The model under review builds one solid part; all positions refer to its coordinate system, in mm. A direction names the side the tool comes from. Coordinates: 2 decimals unless noted, no trailing zeros. Write each loop counter-clockwise with the first axis right and the second up, starting at its lowest first coordinate (ties: lowest second). Pieces come first, ordered by that corner, then holes.
1) For P1, Ø2, axis at y = 13.5, z = -2, coming from the +X side; P2, Ø12, axis at x = 7, z = 12, coming from the -Y side; P3, Ø4, axis at x = 8, z = -10.5, coming from the -Y side; P4, Ø4, axis at y = -8, z = 6, coming from the +X side, all flat-tipped, find the tip position at first contact; note any pin that passes through.
2) For line 1 (Z direction, x = 15, y = 4.5); line 2 (Y direction, x = -4, z = -11.5); line 3 (Z direction, x = -11, y = 13.5), list the stretches that pass through material, from the lowest coordinate up.
3) Mouldability with a two-part tool opening along X and no side actions: class faces 4 (the cylindrical face through (3.226, 8.018, 13.109)), 5 (the flat face through (-4, 17.144, 0)), 6 (the cylindrical face through (-13.4, 8.02, -1.63)) as released by +X, released by -X, zero draft, split by the parting line, or undercut.
4) Add section B-B, the plane z = 5.5. State the section outline as (x, y) points.
5) Machinability: for faces 1 (the cylindrical face through (10.74, -10.72, -2.38)), 2 (the cylindrical face through (-8.96, 8.02, 10.1)), 3 (the cylindrical face through (0.9, 8.02, 2.86)), which of the approach directions +Z, -Z, +X, -X, +Y, -Y give a long, thin tool a straight path to every point of the face, cutting with its end or side? Answer none if there is none.
6) Add section C-C, the plane y = -15. State the section outline as (x, z) points.
7) Add section A-A, the plane x = 0. State the section outline as (y, z) points, then the cut area to 3 significant figures.
from build123d import *

# Parameters (mm, degrees)
SKETCH1_R           = 1.5
BOSS_EXTRUDE1_DEPTH = 9
SKETCH2_R           = 5.5
BOSS_EXTRUDE2_DEPTH = 10
L_EK2_SCALE         = 2


with BuildPart() as part:
    # Sketch1 → Boss-Extrude1 (new body)
    with BuildSketch(Plane(origin=(0, 0, 0), x_dir=(1, 0, 0), z_dir=(0, 1, 0))):
        with BuildLine():
            add(Edge.make_bspline(
                [(-5.065227978, 4.461610195), (-5.526615005, 4.86619147), (-5.830003112, 5.39406146), (-5.975392301, 6.045220165)],
                knots=[0, 0, 0, 0, 0.872429449, 0.872429449, 0.872429449, 0.872429449], degree=3))
            ThreePointArc((-5.065227978, 4.461610195), (-5.560258819, 3.827012132), (-5.976238464, 3.138004752))
            add(Edge.make_bspline(
                [(-7.780961116, 3.42149735), (-7.125870497, 3.507536778), (-6.52429628, 3.413039245), (-5.976238464, 3.138004752)],
                knots=[0.127683247, 0.127683247, 0.127683247, 0.127683247, 1, 1, 1, 1], degree=3))
            ThreePointArc((-7.780961116, 3.42149735), (-7.951879756, 3.00293329), (-8.10030101, 2.575873357))
            add(Edge.make_bspline(
                [(-6.558450277, 1.596630818), (-7.155006493, 1.740452504), (-7.668956737, 2.066866683), (-8.10030101, 2.575873357)],
                knots=[0, 0, 0, 0, 0.872429449, 0.872429449, 0.872429449, 0.872429449], degree=3))
            ThreePointArc((-6.558450277, 1.596630818), (-6.701865893, 0.804669837), (-6.749999881, 0.00126872))
            add(Edge.make_bspline(
                [(-8.479748007, -0.586407486), (-7.939678588, -0.205787566), (-7.363095879, -0.009895497), (-6.749999881, 0.00126872)],
                knots=[0.127683247, 0.127683247, 0.127683247, 0.127683247, 1, 1, 1, 1], degree=3))
            ThreePointArc((-8.479748007, -0.586407486), (-8.436572529, -1.036457408), (-8.369528376, -1.483574994))
            add(Edge.make_bspline(
                [(-6.549210655, -1.634117437), (-7.144272221, -1.784003157), (-7.751044795, -1.733822342), (-8.369528376, -1.483574994)],
                knots=[0, 0, 0, 0, 0.872429449, 0.872429449, 0.872429449, 0.872429449], degree=3))
            ThreePointArc((-6.549210655, -1.634117437), (-6.308156258, -2.402012621), (-5.977417671, -3.13575796))
            add(Edge.make_bspline(
                [(-7.235926822, -4.459973434), (-6.934601997, -3.871968458), (-6.515098947, -3.4305633), (-5.977417671, -3.13575796)],
                knots=[0.127683247, 0.127683247, 0.127683247, 0.127683247, 1, 1, 1, 1], degree=3))
            ThreePointArc((-7.235926822, -4.459973434), (-6.988548208, -4.838408204), (-6.721397655, -5.203154193))
            add(Edge.make_bspline(
                [(-5.039625799, -4.490509081), (-5.496871281, -4.899765193), (-6.0574619, -5.137313564), (-6.721397655, -5.203154193)],
                knots=[0, 0, 0, 0, 0.872429449, 0.872429449, 0.872429449, 0.872429449], degree=3))
            ThreePointArc((-5.039625799, -4.490509081), (-4.469324045, -5.058422935), (-3.835481109, -5.554420281))
            add(Edge.make_bspline(
                [(-4.334442004, -7.311813216), (-4.34089166, -6.651128039), (-4.174571361, -6.065330394), (-3.835481109, -5.554420281)],
                knots=[0.127683247, 0.127683247, 0.127683247, 0.127683247, 1, 1, 1, 1], degree=3))
            ThreePointArc((-4.334442004, -7.311813216), (-3.939531713, -7.53193799), (-3.533475733, -7.730753472))
            add(Edge.make_bspline(
                [(-2.375523406, -6.318179211), (-2.590203375, -6.893050073), (-2.976187484, -7.36390816), (-3.533475733, -7.730753472)],
                knots=[0, 0, 0, 0, 0.872429449, 0.872429449, 0.872429449, 0.872429449], degree=3))
            ThreePointArc((-2.375523406, -6.318179211), (-1.606623554, -6.556009515), (-0.814882047, -6.700631854))
            add(Edge.make_bspline(
                [(-0.439988759, -8.488604708), (-0.752735357, -7.906594341), (-0.877699786, -7.31060339), (-0.814882047, -6.700631854)],
                knots=[0.127683247, 0.127683247, 0.127683247, 0.127683247, 1, 1, 1, 1], degree=3))
            ThreePointArc((-0.439988759, -8.488604708), (0.011984021, -8.499991552), (0.463922896, -8.487330296))
            add(Edge.make_bspline(
                [(0.832782771, -6.698430626), (0.909848909, -7.307220251), (0.786895617, -7.903520141), (0.463922896, -8.487330296)],
                knots=[0, 0, 0, 0, 0.872429449, 0.872429449, 0.872429449, 0.872429449], degree=3))
            ThreePointArc((0.832782771, -6.698430626), (1.624135031, -6.551693323), (2.392396671, -6.311809421))
            add(Edge.make_bspline(
                [(3.555260608, -7.72075916), (3.007863545, -7.350755165), (2.620242233, -6.881105252), (2.392396671, -6.311809421)],
                knots=[0.127683247, 0.127683247, 0.127683247, 0.127683247, 1, 1, 1, 1], degree=3))
            ThreePointArc((3.555260608, -7.72075916), (3.96075436, -7.520799485), (4.355042381, -7.299562032))
            add(Edge.make_bspline(
                [(3.850308451, -5.54415231), (4.201465773, -6.047394331), (4.369710416, -6.632530905), (4.355042381, -7.299562032)],
                knots=[0, 0, 0, 0, 0.872429449, 0.872429449, 0.872429449, 0.872429449], degree=3))
            ThreePointArc((3.850308451, -5.54415231), (4.482823853, -5.046463148), (5.051606144, -4.477027515))
            add(Edge.make_bspline(
                [(6.736042616, -5.184180734), (6.079397157, -5.110946566), (5.517918333, -4.875228826), (5.051606144, -4.477027515)],
                knots=[0.127683247, 0.127683247, 0.127683247, 0.127683247, 1, 1, 1, 1], degree=3))
            ThreePointArc((6.736042616, -5.184180734), (7.002163607, -4.818682892), (7.24847414, -4.439552076))
            add(Edge.make_bspline(
                [(5.985774866, -3.119775513), (6.530577461, -3.402183249), (6.951477219, -3.84210877), (7.24847414, -4.439552076)],
                knots=[0, 0, 0, 0, 0.872429449, 0.872429449, 0.872429449, 0.872429449], degree=3))
            ThreePointArc((5.985774866, -3.119775513), (6.314551754, -2.385149082), (6.553553527, -1.616612559))
            add(Edge.make_bspline(
                [(8.373678438, -1.459968977), (7.758214146, -1.700281702), (7.151505842, -1.75249623), (6.553553527, -1.616612559)],
                knots=[0.127683247, 0.127683247, 0.127683247, 0.127683247, 1, 1, 1, 1], degree=3))
            ThreePointArc((8.373678438, -1.459968977), (8.439461558, -1.01266412), (8.481367828, -0.562494242))
            add(Edge.make_bspline(
                [(6.749972396, 0.019304256), (7.363612555, 0.022427015), (7.940744366, -0.171505818), (8.481367828, -0.562494242)],
                knots=[0, 0, 0, 0, 0.872429449, 0.872429449, 0.872429449, 0.872429449], degree=3))
            ThreePointArc((6.749972396, 0.019304256), (6.699691947, 0.822573894), (6.554160776, 1.614148852))
            add(Edge.make_bspline(
                [(8.093005444, 2.598704077), (7.65971777, 2.099897208), (7.146769547, 1.771712133), (6.554160776, 1.614148852)],
                knots=[0.127683247, 0.127683247, 0.127683247, 0.127683247, 1, 1, 1, 1], degree=3))
            ThreePointArc((8.093005444, 2.598704077), (7.943380571, 3.025343799), (7.771282357, 3.443424244))
            add(Edge.make_bspline(
                [(5.967832596, 3.153961653), (6.509732754, 3.44189952), (7.110882674, 3.53838705), (7.771282357, 3.443424244)],
                knots=[0, 0, 0, 0, 0.872429449, 0.872429449, 0.872429449, 0.872429449], degree=3))
            ThreePointArc((5.967832596, 3.153961653), (5.550013455, 3.841855105), (5.053288778, 4.475128213))
            add(Edge.make_bspline(
                [(5.958322434, 6.062045345), (5.806472362, 5.419014975), (5.504794477, 4.890042598), (5.053288778, 4.475128213)],
                knots=[0.127683247, 0.127683247, 0.127683247, 0.127683247, 1, 1, 1, 1], degree=3))
            ThreePointArc((5.958322434, 6.062045345), (5.627566824, 6.370281912), (5.280889753, 6.660495734))
            add(Edge.make_bspline(
                [(3.818534268, 5.566084444), (4.16455163, 6.072874324), (4.652003458, 6.437678087), (5.280889753, 6.660495734)],
                knots=[0, 0, 0, 0, 0.872429449, 0.872429449, 0.872429449, 0.872429449], degree=3))
            ThreePointArc((3.818534268, 5.566084444), (3.128893766, 5.98101361), (2.394769219, 6.310909632))
            add(Edge.make_bspline(
                [(2.45865956, 8.136645081), (2.623034112, 7.496701718), (2.601737332, 6.888123235), (2.394769219, 6.310909632)],
                knots=[0.127683247, 0.127683247, 0.127683247, 0.127683247, 1, 1, 1, 1], degree=3))
            ThreePointArc((2.45865956, 8.136645081), (2.022545337, 8.25586521), (1.580708948, 8.351727918))
            add(Edge.make_bspline(
                [(0.794455758, 6.703084368), (0.865321915, 7.312626807), (1.127406312, 7.862174657), (1.580708948, 8.351727918)],
                knots=[0, 0, 0, 0, 0.872429449, 0.872429449, 0.872429449, 0.872429449], degree=3))
            ThreePointArc((0.794455758, 6.703084368), (-0.009017778, 6.749993976), (-0.812363108, 6.700937709))
            add(Edge.make_bspline(
                [(-1.604252589, 8.347237485), (-1.161309642, 7.856984441), (-0.897346481, 7.308217849), (-0.812363108, 6.700937709)],
                knots=[0.127683247, 0.127683247, 0.127683247, 0.127683247, 1, 1, 1, 1], degree=3))
            ThreePointArc((-1.604252589, 8.347237485), (-2.045816912, 8.250129282), (-2.481593228, 8.129679886))
            add(Edge.make_bspline(
                [(-2.411622992, 6.304488444), (-2.632142622, 6.877144615), (-2.655466033, 7.485541762), (-2.481593228, 8.129679886)],
                knots=[0, 0, 0, 0, 0.872429449, 0.872429449, 0.872429449, 0.872429449], degree=3))
            ThreePointArc((-2.411622992, 6.304488444), (-3.144863458, 5.972632069), (-3.833392837, 5.555861712))
            add(Edge.make_bspline(
                [(-5.299649804, 6.645578377), (-4.679611352, 6.417326717), (-4.19085903, 6.054087828), (-3.833392837, 5.555861712)],
                knots=[0.127683247, 0.127683247, 0.127683247, 0.127683247, 1, 1, 1, 1], degree=3))
            ThreePointArc((-5.299649804, 6.645578377), (-5.645507162, 6.35438816), (-5.975392301, 6.045220165))
        make_face()
        with Locations(Location((0, 0, 0), (0, 0, 270))):
            Circle(SKETCH1_R, mode=Mode.SUBTRACT)
    extrude(amount=BOSS_EXTRUDE1_DEPTH)

    # Sketch2 → Boss-Extrude2 (add)
    with BuildSketch(Plane.XZ):
        with Locations(Location((0, 0, 0), (0, 0, 90))):
            Circle(SKETCH2_R)
    extrude(amount=BOSS_EXTRUDE2_DEPTH)


with BuildPart() as part_1:
    # Ölçek2: scaled about (0, 0.855834843, 0)
    add(part.part.scale(L_EK2_SCALE).moved(Location((0, -0.855834843, 0))))


solid = part_1.part
Geometry results:
1. P1: stops at x = 13.46
1. P2: stops at y = -20.86
1. P3: stops at y = -0.86
1. P4: stops at x = 10.25
2. line 1: z = -6.94 to -4.11, 0.16 to 3.35
2. line 2: y = -0.86 to 17.14
2. line 3: z = -12.96 to -9.89, -7.83 to 9.65
3. face 4: undercut
3. face 5: zero draft
3. face 6: released by -X
4. outline: (-12.33, -0.86) - (-9.53, -0.86) - (-9.53, -20.86) - (9.53, -20.86) - (9.53, -0.86) - (12.33, -0.86) - (12.33, 17.14) - (-12.33, 17.14) - close
5. face 1: -Y
5. face 2: +Y, -Y
5. face 3: +Y
6. outline: circle Ø22 at (0, 0)
7. outline: (-20.86, -11) - (-0.86, -11) - (-0.86, -13.5) - (17.14, -13.5) - (17.14, -3) - (-0.86, -3) - (-0.86, 3) - (17.14, 3) - (17.14, 17) - (-0.86, 17) - (-0.86, 11) - (-20.86, 11) - close
7. area: 881 mm2
